Build history of the part. All positions in model axes, mm. A direction names the side the tool comes from. Coordinates: 2 decimals unless noted, no trailing zeros. Write each loop counter-clockwise with the first axis right and the second up, starting at its lowest first coordinate (ties: lowest second). Pieces come first, ordered by that corner, then holes.
Autodesk Inventor part; units mm, degrees
ref_plane "YZ Plane" through (0, 0, 0) normal (1, 0, 0) x (0, 1, 0)
ref_plane "XZ Plane" through (0, 0, 0) normal (0, 1, 0) x (-1, 0, 0)
ref_plane "XY Plane" through (0, 0, 0) normal (0, 0, 1) x (1, 0, 0)
sketch "Boceto1" plane through (0, 0, 0) normal (0, 0, 1) x (1, 0, 0)
  line L0 (-3.4064, 0) -> (-1.7032, 2.95)
  line L1 (-1.7032, 2.95) -> (1.7032, 2.95)
  line L2 (1.7032, 2.95) -> (3.4064, 0)
  line L3 (3.4064, 0) -> (1.7032, -2.95)
  line L4 (1.7032, -2.95) -> (-1.7032, -2.95)
  line L5 (-1.7032, -2.95) -> (-3.4064, 0)
  circle A0 centre (0, 0) radius 7.5
extrude "Extrusión1" add sketch "Boceto1" along normal blind 1 contours L0 L1 L2 L3 L4 L5 | A0
sketch "Boceto2" plane through (0, 0, 0) normal (0, 0, -1) x (-1, 0, 0)
  circle A0 centre (0, 0) radius 7.5
  circle A1 centre (0, 0) radius 1.5
  line L0 (1.7032, -2.95) -> (3.4064, 0)
  line L1 (3.4064, 0) -> (1.7032, 2.95)
  line L2 (1.7032, 2.95) -> (-1.7032, 2.95)
  line L3 (-1.7032, 2.95) -> (-3.4064, 0)
  line L4 (-3.4064, 0) -> (-1.7032, -2.95)
  line L5 (-1.7032, -2.95) -> (1.7032, -2.95)
  line L6 (-1.5588, -2.7) -> (-3.1177, 0)
  line L7 (-3.1177, 0) -> (-1.5588, 2.7)
  line L8 (-1.5588, 2.7) -> (1.5588, 2.7)
  line L9 (1.5588, 2.7) -> (3.1177, 0)
  line L10 (3.1177, 0) -> (1.5588, -2.7)
  line L11 (1.5588, -2.7) -> (-1.5588, -2.7)
  dimension "d2" = 0.25
extrude "Extrusión2" add sketch "Boceto2" along normal blind 1.6 contours A1 | L6 L7 L8 L9 L10 L11
properties part number "Tapa_Cabeza_Tornillo"
1. Saw through at D-D on x = 6. List the corners of the cut face in (y, z), plus the area to 3 significant figures.
Computed values:
outline: (-4.5, 0) - (4.5, 0) - (4.5, 1) - (-4.5, 1) - close
area: 9.00 mm2
2. Saw through at B-B on x = 0. List the corners of the cut face in (y, z), plus the area to 3 significant figures.
Computed values:
outline: (-7.5, 0) - (-2.7, 0) - (-2.7, -1.6) - (2.7, -1.6) - (2.7, 0) - (7.5, 0) - (7.5, 1) - (-7.5, 1) - close
area: 23.6 mm2
3. 3-axis set-ups, long thin cutter, end or side, ignore diameter. For faces 1 (the face through (2.35, 1.33, -0.79)), 2 (the face through (0, 2.7, -1)), 3 (the face through (2.327, -1.369, -0.789)), 4 (the face through (-2.35, -1.33, -0.79)), 5 (the face through (-2.327, 1.369, -0.789)): which of +Z, -Z, +X, -X, +Y, -Y reach the whole face in a straight line?
Computed values:
face 1: -Z, +X, +Y
face 2: -Z, +X, -X, +Y
face 3: -Z, +X, -Y
face 4: -Z, -X, -Y
face 5: -Z, -X, +Y
4. Saw through at C-C on y = -2. List the corners of the cut face in (x, z).
Computed values:
outline: (-7.23, 0) - (-1.96, 0) - (-1.96, -1.6) - (1.96, -1.6) - (1.96, 0) - (7.23, 0) - (7.23, 1) - (-7.23, 1) - close
5. Probe line 1 along Z through (x, y) = (-6, 3.5); line 2 along Y through (x, z) = (-0.75, 0.5); line 3 along Y through (x, z) = (-2.5, -0.7). List the from-to ranges inside material, lowest first.
Computed values:
line 1: z = 0 to 1
line 2: y = -7.46 to 7.46
line 3: y = -1.07 to 1.07
6. Saw through at A-A on z = -0.9. List the corners of the cut face in (x, y), plus the area to 3 significant figures.
Computed values:
outline: (-3.12, 0) - (-1.56, -2.7) - (1.56, -2.7) - (3.12, 0) - (1.56, 2.7) - (-1.56, 2.7) - close
area: 25.3 mm2
7. Flat gauge pins, fed straight in: pin 1 (0.5 mm diameter, centred on x = 0.5, z = -0.5, fed in from -Y); pin 2 (0.8 mm diameter, centred on x = -0.5, z = -1, fed in from +Y). Where does each tip first touch, or does it go through?
Computed values:
pin 1: stops at y = -2.7
pin 2: stops at y = 2.7
